Input: part model. Units: mm. Frame: model coordinates. Round coordinates to 2 decimals unless told otherwise and drop trailing zeros. Loops run counter-clockwise (first coordinate to the right, second up) from the corner with the lowest first, then second, coordinate; pieces in that order, holes last. Notation, with made-up numbers: M 57,-6 L 114,-6 A14 cw 114,19 Z; hole C -27,-7 d2. An arc over 180 degrees is marked long. Return JSON: item names as keys, results as strings. Group by question number.
1) Material intervals for line 1 (X direction, y = -83.82, z = 2.35); line 2 (Y direction, x = 31, z = 0.9); line 3 (X direction, y = -61.5, z = 0.9), sorted ascending. Write a range as from..to.
2) Section B-B (z = 1.9). Count the separate pieces of the cut face and the enclosed holes in it, plus the area to 3 significant figures.
3) Contact query for flat-ended pins moving along their axis: P1, Ø2.5, axis at x = -60.198, y = -83.82, coming from the +Z side; P2, Ø1, axis at x = 7, z = 2, coming from the -Y side; P3, Ø1.6, axis at x = 19.5, z = 1, coming from the -Y side; P4, Ø1, axis at y = -144, z = 1, coming from the -X side. Output: stop coordinate, or through.
4) Section A-A (y = -48.26). Output: boundary loops of the cut face in (x, z) (3 decimals).
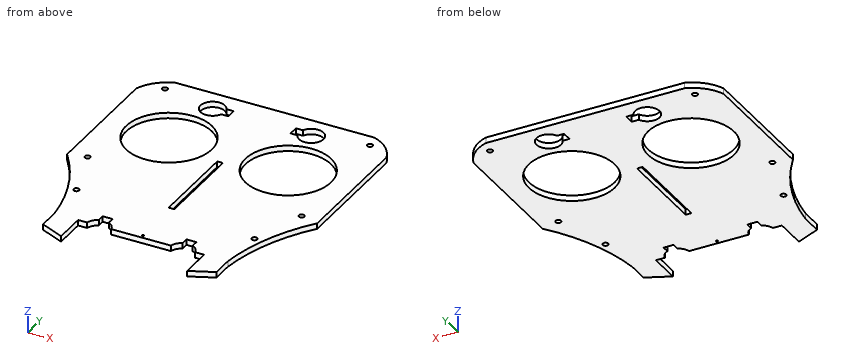
from build123d import *

# Parameters (mm, degrees)
SKETCH1_W                           = 140.716
SKETCH1_H                           = 139.7
MAIN_BODY_DEPTH                     = 3.175
SKETCH2_R                           = 24.13
CUTS_FOR_EYES_AND_MOTORS_DEPTH      = 4.175
SKETCH4_W                           = 3.2258
SKETCH4_H                           = 50.8
CUT_FOR_NOSE_DEPTH                  = 4.175
CUT_FOR_ROUNDED_FACE_FEATURES_DEPTH = 4.175
SKETCH12_R                          = 1.524
HOLES_FOR_SPACERS_DEPTH             = 4.175
BOSS_EXTRUDE1_DEPTH                 = 3.175
CUT_EXTRUDE1_DEPTH                  = 4.175
SKETCH16_R                          = 0.508
CUT_EXTRUDE2_DEPTH                  = 4.175


with BuildPart() as part:
    # Sketch1 → main body (new body)
    with BuildSketch(Plane.XY):
        with Locations((0, -69.85)):
            Rectangle(SKETCH1_W, SKETCH1_H)
    extrude(amount=MAIN_BODY_DEPTH)

    # Sketch2 → cuts for eyes and motors (cut, through all)
    with BuildSketch(Plane.XY.offset(3.175)):
        with Locations((-33.528, -48.26)):
            Circle(SKETCH2_R)
        with BuildLine():
            Line((-17.500552949, -13.319125673), (-17.500552949, -10.525125673))
            Line((-17.500552949, -10.525125673), (-21.496618579, -10.525125673))
            ThreePointArc((-21.496618579, -10.525125673), (-34.59452735, -13.425551762), (-21.451292126, -16.113125673))
            Line((-21.451292126, -16.113125673), (-17.500552949, -16.113125673))
            Line((-17.500552949, -16.113125673), (-17.500552949, -13.319125673))
        make_face()
    cuts_for_eyes_and_motors = extrude(amount=-CUTS_FOR_EYES_AND_MOTORS_DEPTH, mode=Mode.SUBTRACT)

    # Sketch4 → cut for nose (cut, through all)
    with BuildSketch(Plane.XY.offset(3.175)):
        with Locations((0, -82.55)):
            Rectangle(SKETCH4_W, SKETCH4_H)
    extrude(amount=-CUT_FOR_NOSE_DEPTH, mode=Mode.SUBTRACT)

    # Mirror1: cuts for eyes and motors across plane
    add(cuts_for_eyes_and_motors.mirror(Plane(origin=(0, 0, 0), x_dir=(0, 0, 1), z_dir=(1, 0, 0))), mode=Mode.SUBTRACT)

    # Sketch11 → cut for rounded face features (cut, through all)
    with BuildSketch(Plane.XY.offset(3.175)):
        with BuildLine():
            Line((-70.358, -139.7), (-70.358, -86.36))
            ThreePointArc((-70.358, -86.36), (-55.943359781, -111.56490753), (-48.768, -139.7))
            Line((-48.768, -139.7), (-70.358, -139.7))
        make_face()
        with BuildLine():
            Line((-70.358, 0), (-70.358, -13.97))
            ThreePointArc((-70.358, -13.97), (-64.724440046, -5.321180316), (-55.88, 0))
            Line((-55.88, 0), (-70.358, 0))
        make_face()
    cut_for_rounded_face_features = extrude(amount=-CUT_FOR_ROUNDED_FACE_FEATURES_DEPTH, mode=Mode.SUBTRACT)

    # mirror of rounded feature: cut for rounded face features across plane
    add(cut_for_rounded_face_features.mirror(Plane(origin=(0, 0, 0), x_dir=(0, 0, 1), z_dir=(1, 0, 0))), mode=Mode.SUBTRACT)

    # Sketch12 → holes for spacers (cut, through all)
    with BuildSketch(Plane.XY.offset(3.175)):
        with Locations((-57.658, -7.62)):
            Circle(SKETCH12_R)
        with Locations((-60.198, -83.82)):
            Circle(SKETCH12_R)
        with Locations((-50.038, -114.3)):
            Circle(SKETCH12_R)
    holes_for_spacers = extrude(amount=-HOLES_FOR_SPACERS_DEPTH, mode=Mode.SUBTRACT)

    # mirror of spacer hole: holes for spacers across plane
    add(holes_for_spacers.mirror(Plane(origin=(0, 0, 0), x_dir=(0, 0, 1), z_dir=(1, 0, 0))), mode=Mode.SUBTRACT)

    # Sketch14 → Boss-Extrude1 (add)
    with BuildSketch(Plane.XY.offset(3.175)):
        Polygon((-48.768, -139.7), (-35.433, -139.7), (-35.433, -157.48), (-48.768, -151.596070028), align=None)
    boss_extrude1 = extrude(amount=-BOSS_EXTRUDE1_DEPTH)

    # Mirror3: Boss-Extrude1 across plane
    add(boss_extrude1.mirror(Plane(origin=(0, 0, 0), x_dir=(0, 0, 1), z_dir=(1, 0, 0))))

    # Sketch15 → Cut-Extrude1 (cut, through all)
    with BuildSketch(Plane.XY.offset(3.175)):
        with BuildLine():
            Line((-23.622, -130.7846), (-26.416, -130.7846))
            Line((-26.416, -130.7846), (-26.416, -134.78066563))
            ThreePointArc((-26.416, -134.78066563), (-23.515573911, -147.878574401), (-20.828, -134.735339177))
            Line((-20.828, -134.735339177), (-20.828, -130.7846))
            Line((-20.828, -130.7846), (-23.622, -130.7846))
        make_face()
        with BuildLine():
            Line((23.5204, -130.7846), (20.7264, -130.7846))
            Line((20.7264, -130.7846), (20.7264, -134.78066563))
            ThreePointArc((20.7264, -134.78066563), (23.626826089, -147.878574401), (26.3144, -134.735339177))
            Line((26.3144, -134.735339177), (26.3144, -130.7846))
            Line((26.3144, -130.7846), (23.5204, -130.7846))
        make_face()
    extrude(amount=-CUT_EXTRUDE1_DEPTH, mode=Mode.SUBTRACT)

    # Sketch16 → Cut-Extrude2 (cut, through all)
    with BuildSketch(Plane.XY.offset(3.175)):
        with Locations((0, -137.668)):
            Circle(SKETCH16_R)
    extrude(amount=-CUT_EXTRUDE2_DEPTH, mode=Mode.SUBTRACT)


solid = part.part
Returned:
{
 "1": {"line 1": "x = -70.36..-61.72, -58.67..-1.61, 1.61..58.67, 61.72..70.36", "line 2": "y = -139.7..-72.26, -24.26..-19.4, -7.34..0", "line 3": "x = -70.36..-53.7, -13.35..-1.61, 1.61..13.35, 53.7..70.36"},
 "2": {"separate pieces": "1", "enclosed holes": "12", "area": "14,100 mm^2"},
 "3": {"P1": "passes through", "P2": "stops at y = -139.7", "P3": "stops at y = -136.19", "P4": "stops at x = -48.77"},
 "4": {"outline": "M -70.358,0 L -57.658,0 L -57.658,3.175 L -70.358,3.175 Z; M -9.398,0 L 9.398,0 L 9.398,3.175 L -9.398,3.175 Z; M 57.658,0 L 70.358,0 L 70.358,3.175 L 57.658,3.175 Z"}
}
